Drawing for the job (mm, zero at the part's lowest x, y, z). Give positions to 0.01 mm unless a question says otherwise; leave off trailing zeros. Loops run counter-clockwise (first coordinate to the right, second up) from the corner with the lowest first, then second, coordinate; pieces in that order, holes last.
1) Band-saw the part on C-C on x = 5.5. List the corners of the cut face in (y, z) (1 decimal), then the cut area to 3 significant figures.
2) Wall check: line 1 (X direction, y = 10, z = 15.5); line 2 (X direction, y = 2.75, z = 7.5); line 3 (Y direction, x = 6, z = 11.5). Give the ranges that are in metal, low to high.
3) Band-saw the part on A-A on z = 16. List the corners of the cut face in (x, y), then the cut area to 3 significant figures.
4) Band-saw the part on B-B on y = 15. List the corners of the cut face in (x, z), then the cut area to 3 significant figures.
5) Flat gauge pins, fed straight in: P1, Ø8, axis at x = 10.5, z = 7, coming from the +Y side; P2, Ø2, axis at x = 6.5, z = 16, coming from the +Y side; P3, Ø8, axis at y = 2, z = 3.5, coming from the -X side (1 decimal). Where does each tip first touch, or does it go through?
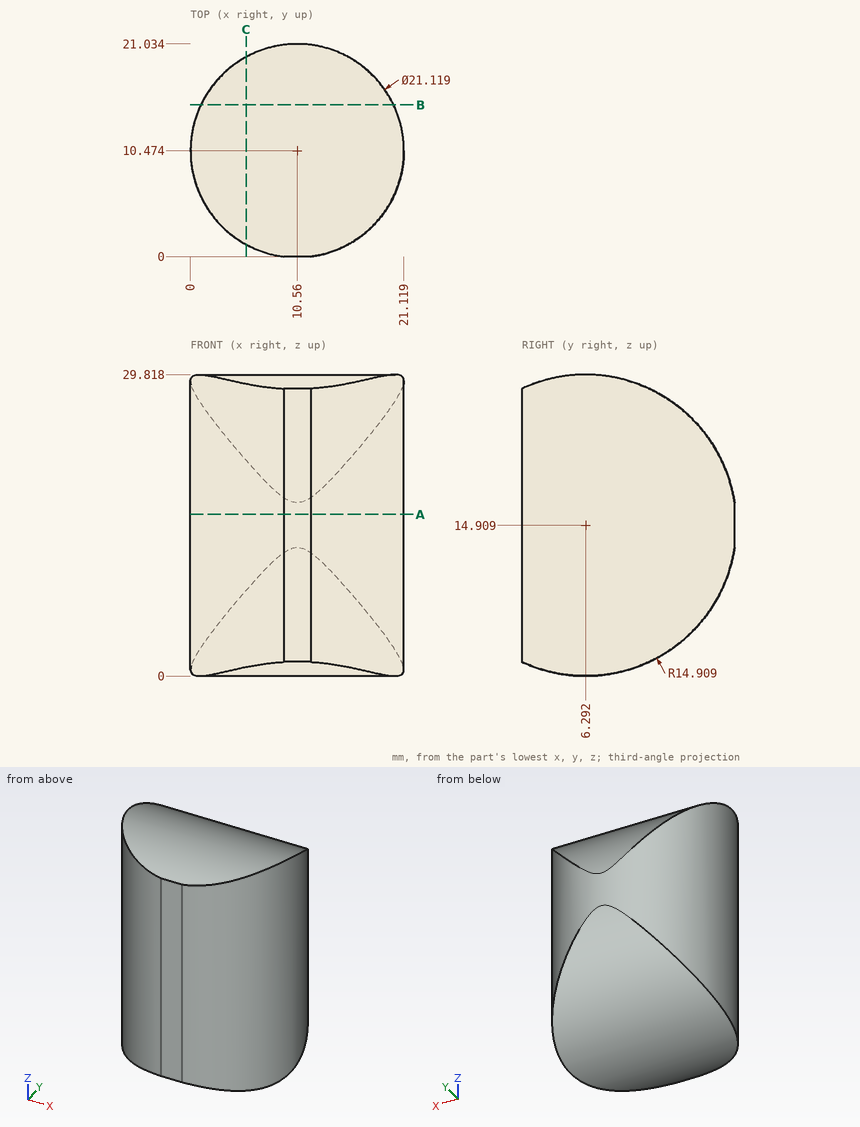
Findings below:
1. outline: (1.2, 0.9) arc R14.9 ccw to (19.7, 8.5) - (19.7, 21.3) arc R14.9 ccw to (1.2, 28.9) - close
1. area: 485 mm2
2. line 1: x = 0.01 to 21.11
2. line 2: x = 3.36 to 17.76
2. line 3: y = 0.95 to 20
3. outline: (9.22, 0) - (11.9, 0) arc R10.56 ccw (long way) to start
3. area: 350 mm2
4. outline: (1.02, 2.81) - (20.1, 2.81) - (20.1, 27.01) - (1.02, 27.01) - close
4. area: 462 mm2
5. P1: stops at y = 20.68
5. P2: stops at y = 20.58
5. P3: stops at x = 1
